```python
from build123d import *

# Parameters (mm, degrees)
SKETCH_1_R          = 13
EXTRUDE_1_DEPTH     = 4
SKETCH_2_R          = 12
SKETCH_2_R_2        = 10.075
EXTRUDE_2_DEPTH     = 5.2
SKETCH_3_W          = 10
SKETCH_3_H          = 1.5
CUT_EXTRUDE_1_DEPTH = 2.5


with BuildPart() as part:
    # 스케치1 → 보스-돌출1 (new body)
    with BuildSketch(Plane.XY):
        Circle(SKETCH_1_R)
    extrude(amount=EXTRUDE_1_DEPTH)

    # 스케치2 → 보스-돌출2 (add)
    with BuildSketch(Plane.XY):
        Circle(SKETCH_2_R)
        Circle(SKETCH_2_R_2, mode=Mode.SUBTRACT)
    extrude(amount=-EXTRUDE_2_DEPTH)

    # 스케치3 → 컷-돌출1 (cut)
    with BuildSketch(Plane.XY.offset(4)):
        Rectangle(SKETCH_3_W, SKETCH_3_H)
    extrude(amount=-CUT_EXTRUDE_1_DEPTH, mode=Mode.SUBTRACT)


solid = part.part
```
The listing builds one solid part. Answer for the finished solid, in the listing's coordinates (mm). A direction names the side the tool comes from. Give positions to 0.01 mm unless a question says otherwise; leave off trailing zeros. Order: outer loops, then holes, each group sorted by start corner. A loop starts at its lowest first (then second) coordinate and runs counter-clockwise, first axis right, second up.
1) Consider line 1 along X through (y, z) = (-0.25, -1.75); line 2 along Y through (x, z) = (0, -2.3) (3 decimals); line 3 along Z through (x, y) = (-1, 5.75). Determine where each line is inside the solid, lowest interval first.
Reported:
line 1: x = -12 to -10.07, 10.07 to 12
line 2: y = -12 to -10.075, 10.075 to 12
line 3: z = 0 to 4
2) For faces 1 (the face through (5, 0, 3)), 2 (the face through (9, -9, 0)), 3 (the face through (-10.316, -7.91, 1.972)), determine the directions among +Z, -Z, +X, -X, +Y, -Y from which every point of the face is accessible in a straight line to the end or side of a thin tool.
Reported:
face 1: +Z
face 2: -Z
face 3: +Z, -Z
3) Find section B-B on z = 3.25. Write down the section's boundary in (x, y), then the cut area to 3 significant figures.
Reported:
outline: circle Ø26 at (0, 0); hole (-5, -0.75) - (5, -0.75) - (5, 0.75) - (-5, 0.75) - close
area: 516 mm2
4) Find section C-C on y = 7.5. Write down the section's boundary in (x, z).
Reported:
outline: (-10.62, 0) - (-9.37, 0) - (-9.37, -5.2) - (-6.73, -5.2) - (-6.73, 0) - (6.73, 0) - (6.73, -5.2) - (9.37, -5.2) - (9.37, 0) - (10.62, 0) - (10.62, 4) - (-10.62, 4) - close
5) Determine the mould class of faces 4 (the face through (-3, 10, -5.2)), 5 (the face through (9.307, -3.859, -2.564)), 6 (the face through (-11.99, 0.53, -2.56)) for opening direction X: pulls with the +X half, pulls with the -X half, needs draft (parallel to the pull), parting line crosses it, or undercut.
Reported:
face 4: needs draft
face 5: undercut
face 6: parting line crosses it
6) Given P1, Ø1.2, axis at x = -2, y = 0, coming from the +Z side; P2, Ø3, axis at x = -2, z = 2, coming from the -Y side; P3, Ø5, axis at y = 0, z = -3.5, coming from the +X side, each flat-ended and moving along its own axis, determine where each tip first touches the part or whether it passes through.
Reported:
P1: stops at z = 1.5
P2: stops at y = -12.99
P3: stops at x = 12
7) Find section D-D on z = -2. Write down the section's boundary in (x, y) (3 decimals).
Reported:
outline: circle Ø24 at (0, 0); hole circle Ø20.15 at (0, 0)
8) Find section A-A on x = 0. Write down the section's boundary in (y, z) (3 decimals).
Reported:
outline: (-13, 0) - (-12, 0) - (-12, -5.2) - (-10.075, -5.2) - (-10.075, 0) - (10.075, 0) - (10.075, -5.2) - (12, -5.2) - (12, 0) - (13, 0) - (13, 4) - (0.75, 4) - (0.75, 1.5) - (-0.75, 1.5) - (-0.75, 4) - (-13, 4) - close
